Input: part model. Units: mm. Frame: model coordinates. Coordinates: 2 decimals unless noted, no trailing zeros. Write each loop counter-clockwise with the first axis right and the second up, starting at its lowest first coordinate (ties: lowest second). Pieces come first, ordered by that corner, then holes. Notation, with made-up numbers: (-11.5, 27.5) - (32.5, 27.5) arc R21 ccw to (32.5, 64.5) - close; hole circle Ø4 at (49, 37.25). An arc over 180 degrees is marked (long way). Use a Markdown table: item, result. Add a question column.
Q1. Material intervals for probe 1 along X at (y, z) = (0.95, -16.5); probe 2 along Z at (x, y) = (192.5, 1.3); probe 3 along X at (y, z) = (0.65, -7.5), sorted ascending. Write a range as from..to.
Q2. Section query A-A (x = -94.5). Return the cut outline in (y, z), then the cut area to 3 significant figures.
Q3. Pin query (flat end, axial travel): P1, Ø3.5, axis at x = -192.5, z = 16, coming from the -Y side. Return the tip coordinate at first contact, or that it passes through.
Q4. Section query B-B (y = 1.25). Give the number of separate pieces and of enclosed holes in the cut face, then the cut area to 3 significant figures.
from build123d import *

# Parameters (mm, degrees)
SKIZZE1_W                       = 393
SKIZZE1_H                       = 40
AUFSATZ_LINEAR_AUSTRAGEN1_DEPTH = 1.5
SKIZZE2_R                       = 1.6
SCHNITT_LINEAR_AUSTRAGEN1_DEPTH = 198.520884972
FASE1_SIZE                      = 1
SCHNITT_LINEAR_AUSTRAGEN2_DEPTH = 198.520884972


with BuildPart() as part:
    # Skizze1 → Aufsatz-Linear austragen1 (new body)
    with BuildSketch(Plane(origin=(0, 0, 0), x_dir=(1, 0, 0), z_dir=(0, 1, 0))):
        Rectangle(SKIZZE1_W, SKIZZE1_H)
    extrude(amount=AUFSATZ_LINEAR_AUSTRAGEN1_DEPTH)

    # Skizze2 → Schnitt-Linear austragen1 (cut, through all)
    with BuildSketch(Plane(origin=(0, 1.5, 0), x_dir=(1, 0, 0), z_dir=(0, 1, 0))):
        with Locations(Location((-192.5, 16, 0), (0, 0, 270))):
            Circle(SKIZZE2_R)
        with Locations(Location((-192.5, -16, 0), (0, 0, 270))):
            Circle(SKIZZE2_R)
        with Locations(Location((192.5, -16, 0), (0, 0, 270))):
            Circle(SKIZZE2_R)
        with Locations(Location((192.5, 16, 0), (0, 0, 270))):
            Circle(SKIZZE2_R)
        with Locations(Location((44.5, -15, 0), (0, 0, 270))):
            Circle(SKIZZE2_R)
        with BuildLine():
            ThreePointArc((-16.400011, 8.5), (-16.86864015, 9.63137085), (-18.000011, 10.1))
            Line((-18.000011, 10.1), (-18.000011, 6.9))
            ThreePointArc((-18.000011, 6.9), (-16.86864015, 7.36862915), (-16.400011, 8.5))
        make_face()
        with BuildLine():
            Line((-18.000011, 6.9), (-18.000011, 10.1))
            ThreePointArc((-18.000011, 10.1), (-19.600011, 8.5), (-18.000011, 6.9))
        make_face()
        with BuildLine():
            ThreePointArc((145.099964038, 8.589999773), (144.631340773, 9.721364737), (143.499980683, 10.189999773))
            Line((143.499980683, 10.189999773), (143.499947392, 6.989999773))
            ThreePointArc((143.499947392, 6.989999773), (144.631329002, 7.458623038), (145.099964038, 8.589999773))
        make_face()
        with BuildLine():
            Line((143.499947392, 6.989999773), (143.499980683, 10.189999773))
            ThreePointArc((143.499980683, 10.189999773), (141.899964038, 8.590016418), (143.499947392, 6.989999773))
        make_face()
        with Locations(Location((-31.5, -15, 0), (0, 0, 270))):
            Circle(SKIZZE2_R)
    extrude(amount=-SCHNITT_LINEAR_AUSTRAGEN1_DEPTH, mode=Mode.SUBTRACT)

    # Fase1
    fase1_edges = [part.edges().sort_by_distance(p)[0] for p in [
        (44.5, 0, 13.4),
        (192.5, 0, -17.6),
        (192.5, 0, 14.4),
        (-192.5, 0, 14.4),
        (-18.000011, 0, -10.1),
        (143.499947392, 0, -6.989999773),
        (-31.5, 0, 13.4),
        (-192.5, 0, -17.6),
    ]]
    chamfer(fase1_edges, length=FASE1_SIZE)

    # Skizze3 → Schnitt-Linear austragen2 (cut, through all)
    with BuildSketch(Plane.XZ):
        with BuildLine():
            Line((-64.700005979, -2.35700022), (-62.000005979, -2.35700022))
            ThreePointArc((-62.000005979, -2.35700022), (-60.750005979, -3.60700022), (-62.000005979, -4.85700022))
            Line((-62.000005979, -4.85700022), (-64.700005979, -4.85700022))
            ThreePointArc((-64.700005979, -4.85700022), (-65.950005979, -3.60700022), (-64.700005979, -2.35700022))
        make_face()
        with BuildLine():
            Line((-111.800007059, 2.092999135), (-125.200007059, 2.093000306))
            ThreePointArc((-125.200007059, 2.093000306), (-126.013179849, 1.756173213), (-126.350007159, 0.943000513))
            Line((-126.350007159, 0.943000513), (-126.350007376, -1.535427197))
            ThreePointArc((-126.350007376, -1.535427197), (-126.125055687, -2.21864441), (-125.538206197, -2.634573128))
            Line((-125.538206197, -2.634573128), (-125.004483233, -2.79879563))
            Line((-125.004483233, -2.79879563), (-124.152708289, -3.766721872))
            ThreePointArc((-124.152708289, -3.766721872), (-123.763106884, -4.054897814), (-123.289387767, -4.156999861))
            Line((-123.289387767, -4.156999861), (-113.710627438, -4.157000698))
            ThreePointArc((-113.710627438, -4.157000698), (-113.236908304, -4.054898732), (-112.847306849, -3.766722856))
            Line((-112.847306849, -3.766722856), (-111.995531741, -2.798796767))
            Line((-111.995531741, -2.798796767), (-111.461808748, -2.634574359))
            ThreePointArc((-111.461808748, -2.634574359), (-110.874959185, -2.218645743), (-110.650007376, -1.535428569))
            Line((-110.650007376, -1.535428569), (-110.650007159, 0.942999034))
            ThreePointArc((-110.650007159, 0.942999034), (-110.98683429, 1.756171862), (-111.800007059, 2.092999135))
        make_face()
        with BuildLine():
            Line((-101.915250235, 3.595995958), (-90.084765307, 3.595995958))
            ThreePointArc((-90.084765307, 3.595995958), (-88.918039118, 3.112722147), (-88.434765307, 1.945995958))
            Line((-88.434765307, 1.945995958), (-88.434765307, -2.510004042))
            ThreePointArc((-88.434765307, -2.510004042), (-88.918039118, -3.676730231), (-90.084765307, -4.160004042))
            Line((-90.084765307, -4.160004042), (-101.915250235, -4.160004042))
            ThreePointArc((-101.915250235, -4.160004042), (-103.081976424, -3.676730231), (-103.565250235, -2.510004042))
            Line((-103.565250235, -2.510004042), (-103.565250235, 1.945995958))
            ThreePointArc((-103.565250235, 1.945995958), (-103.081976424, 3.112722147), (-101.915250235, 3.595995958))
        make_face()
        with BuildLine():
            Line((-79.224953939, -0.821999997), (-72.774953939, -0.821999997))
            ThreePointArc((-72.774953939, -0.821999997), (-71.643582904, -1.290629498), (-71.174953542, -2.42200059))
            Line((-71.174953542, -2.42200059), (-71.174954106, -3.082000561))
            ThreePointArc((-71.174954106, -3.082000561), (-71.643583256, -4.213371411), (-72.774954106, -4.682000561))
            Line((-72.774954106, -4.682000561), (-79.224954215, -4.681999997))
            ThreePointArc((-79.224954215, -4.681999997), (-80.356325086, -4.21337078), (-80.824954106, -3.081999827))
            Line((-80.824954106, -3.081999827), (-80.824954106, -2.422000164))
            ThreePointArc((-80.824954106, -2.422000164), (-80.356324907, -1.290629196), (-79.224953939, -0.821999997))
        make_face()
    extrude(amount=-SCHNITT_LINEAR_AUSTRAGEN2_DEPTH, mode=Mode.SUBTRACT)


solid = part.part
Values follow:
| question | item | result |
|---|---|---|
| 1 | probe 1 | -196.5..-194.07, -190.93..190.93, 194.07..196.5 |
| 1 | probe 2 | -20..-17.6, -14.4..14.4, 17.6..20 |
| 1 | probe 3 | -196.5..-19.67, -16.33..141.88, 145.12..196.5 |
| 2 | outline | (0, -20) - (1.5, -20) - (1.5, -4.16) - (0, -4.16) - close; (0, 3.6) - (1.5, 3.6) - (1.5, 20) - (0, 20) - close |
| 2 | area | 48.4 mm2 |
| 3 | P1 | y = 0.85 |
| 4 | separate pieces | 1 |
| 4 | enclosed holes | 12 |
| 4 | area | 15,400 mm2 |
